Autodesk Inventor part; units mm, degrees
ref_plane "YZ Plane" through (0, 0, 0) normal (1, 0, 0) x (0, 1, 0)
ref_plane "XZ Plane" through (0, 0, 0) normal (0, 1, 0) x (-1, 0, 0)
ref_plane "XY Plane" through (0, 0, 0) normal (0, 0, 1) x (1, 0, 0)
sketch "Sketch1" plane through (0, 0, 0) normal (0, 0, 1) x (1, 0, 0)
  line L0 (-12.1708, 16.0073) -> (13.2292, 16.0073)
  line L1 (13.2292, 16.0073) -> (13.2292, -34.7927)
  line L2 (13.2292, -34.7927) -> (-12.1708, -34.7927)
  line L3 (-12.1708, -34.7927) -> (-12.1708, 16.0073)
  line L4 (11.9592, 14.7373) -> (-10.9008, 14.7373)
  line L5 (-10.9008, 14.7373) -> (-10.9008, -33.5227)
  line L6 (-10.9008, -33.5227) -> (11.9592, -33.5227)
  line L7 (11.9592, -33.5227) -> (11.9592, 14.7373)
  point P0 (0, 0)
  dimension "d0" = 25.4
  dimension "d1" = 50.8
  dimension "d2" = 1.27
extrude "Extrusion1" add sketch "Sketch1" along normal blind 152.4
sketch "Sketch2" plane through (-12.1708, 16.0073, 0) normal (0, 1, 0) x (1, 0, 0)
  circle A0 centre (12.7, -12.7) radius 1.7272
  line L0 (25.4, 0) -> (0, 0)
  line L1 (0, 0) -> (0, -152.4)
  point P0 (12.1708, 0)
  dimension "d5" = 3.4544
  dimension "d6" = 12.7
  dimension "d7" = 12.7
extrude "Extrusion2" cut sketch "Sketch2" against normal through all
pattern_linear "Rectangular Pattern1" count 6 spacing 25.4 along (0, 0, 1) of "Extrusion2"
sketch "Sketch3" plane through (13.2292, -34.7927, 0) normal (1, 0, 0) x (0, 0, -1)
  circle A0 centre (-127.1277, 25.5483) radius 14.2875
  line L0 (-152.5277, 50.9483) -> (-127.1277, 25.5483) construction
  point P0 (0, 34.7927)
  dimension "d15" = 25.4
  dimension "d16" = 25.4
  dimension "d17" = 28.575
extrude "Extrusion3" cut sketch "Sketch3" against normal through all
equation "\"d3\" = d13"
equation "\"d13\" = 152.4"
properties part number "VerseFrame 6in w Bearing Hole"
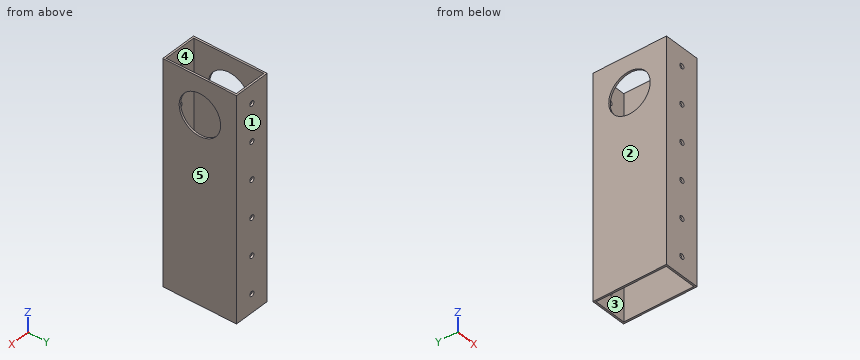
The model under review builds one solid part; all positions refer to its coordinate system, in mm. Face numbers are marked on the shaded views. A direction names the side the tool comes from. Round coordinates to 2 decimals unless told otherwise and drop trailing zeros. Write each loop counter-clockwise with the first axis right and the second up, starting at its lowest first coordinate (ties: lowest second). Pieces come first, ordered by that corner, then holes. Notation, with made-up numbers: M 2.5,2 L 55.5,2 A21 ccw 55.5,22 Z; hole C 61.5,67 d3. An arc over 180 degrees is marked long. Use a Markdown table: item, result. Add a question column.
Q1. Machinability: for the marked faces 4 and 5, which of the approach directions +Z, -Z, +X, -X, +Y, -Y give a long, thin tool a straight path to every point of the face, cutting with its end or side? Answer none if there is none.
Q2. We need section B-B, the plane x = -9.5. State the section outline as (y, z) points, plus the area to 3 significant figures.
Q3. We need section A-A, the plane z = 88.9. State the section outline as (x, y) points.
Q4. We need section D-D, the plane z = 139.7. State the section outline as (x, y) points, plus the area to 3 significant figures.
Q5. To check wall thickness, follow line 1 (Y direction, x = 8, z = 141); line 2 (X direction, y = -34.4, z = 63.5); line 3 (X direction, y = -29, z = 14.5). State the ranges of each line that lie inside material, in increasing order.
Q6. The part is to be moulded in two halves that separate along Y. For the marked faces 1, 2 and 3, say which applies: pulls with the +Y half, pulls with the -Y half, needs draft (parallel to the pull), parting line crosses it, or undercut.
Q7. Insertion check: pin 1 (3 mm diameter, centred on x = 0.53, z = 63.5, fed in from +Y). The pin has a flat end and moves straight along its axis. Give the tip position at first contact, or say it passes through.
Q8. We need section C-C, the plane y = -25. State the section outline as (x, z) points, plus the area to 3 significant figures.
Findings below:
| question | item | result |
|---|---|---|
| 1 | face 4 | +Z, -Z |
| 1 | face 5 | +Z, -Z, +X, +Y, -Y |
| 2 | outline | M -34.79,0 L -33.52,0 L -33.52,152.4 L -34.79,152.4 Z; M 14.74,0 L 16.01,0 L 16.01,152.4 L 14.74,152.4 Z |
| 2 | area | 387 mm² |
| 3 | outline | M -12.17,-34.79 L -1.2,-34.79 L -1.2,-33.52 L -10.9,-33.52 L -10.9,14.74 L -1.2,14.74 L -1.2,16.01 L -12.17,16.01 Z; M 2.26,-34.79 L 13.23,-34.79 L 13.23,16.01 L 2.26,16.01 L 2.26,14.74 L 11.96,14.74 L 11.96,-33.52 L 2.26,-33.52 Z |
| 4 | outline | M -12.17,-34.79 L -1.2,-34.79 L -1.2,-33.52 L -10.9,-33.52 L -10.9,-16.03 L -12.17,-16.03 Z; M -12.17,-2.46 L -10.9,-2.46 L -10.9,14.74 L -1.2,14.74 L -1.2,16.01 L -12.17,16.01 Z; M 2.26,-34.79 L 13.23,-34.79 L 13.23,-16.03 L 11.96,-16.03 L 11.96,-33.52 L 2.26,-33.52 Z; M 2.26,14.74 L 11.96,14.74 L 11.96,-2.46 L 13.23,-2.46 L 13.23,16.01 L 2.26,16.01 Z |
| 4 | area | 144 mm² |
| 5 | line 1 | y = -34.79 to -33.52, 14.74 to 16.01 |
| 5 | line 2 | x = -12.17 to -1.2, 2.26 to 13.23 |
| 5 | line 3 | x = -12.17 to -10.9, 11.96 to 13.23 |
| 6 | face 1 | pulls with the +Y half |
| 6 | face 2 | needs draft |
| 6 | face 3 | undercut |
| 7 | pin 1 | passes through |
| 8 | outline | M -12.17,0 L -10.9,0 L -10.9,152.4 L -12.17,152.4 Z; M 11.96,0 L 13.23,0 L 13.23,152.4 L 11.96,152.4 Z |
| 8 | area | 387 mm² |
